The model under review builds one solid part; all positions refer to its coordinate system, in mm. Face numbers are marked on the shaded views. Coordinates: 2 decimals unless noted, no trailing zeros. Loops run counter-clockwise (first coordinate to the right, second up) from the corner with the lowest first, then second, coordinate; pieces in that order, holes last. Notation, with made-up numbers: M 32.5,-35 L 68.5,-35 A14 cw 68.5,-11 Z; hole C 2,38 d2. An arc over 180 degrees is marked long. Use one line per item in the form item = value.
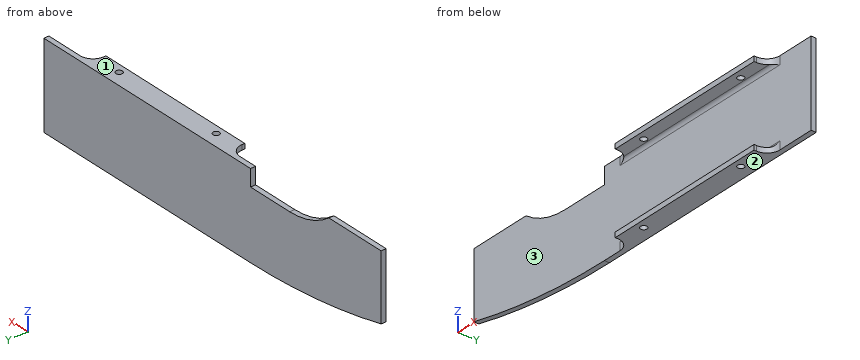
```python
from build123d import *

# Parameters (mm, degrees)
SKETCH1_W           = 132.917449813
SKETCH1_H           = 12
SKETCH1_R           = 2.55
BOSS_EXTRUDE1_DEPTH = 4
SKETCH2_W           = 197.917449813
SKETCH2_H           = 67
BOSS_EXTRUDE2_DEPTH = 4
BOSS_EXTRUDE3_START = 4
SKETCH3_W           = 132.917449813
SKETCH3_H           = 12
SKETCH3_R           = 2.55
BOSS_EXTRUDE3_DEPTH = 4
FILLET1_R           = 10
FILLET2_R           = 2.5
BOSS_EXTRUDE4_DEPTH = 4


with BuildPart() as part:
    # Sketch1 → Boss-Extrude1 (new body)
    with BuildSketch(Plane.XY):
        with Locations((-116.458724907, 49.8)):
            Rectangle(SKETCH1_W, SKETCH1_H)
        with Locations((-162.917449813, 49.8)):
            Circle(SKETCH1_R, mode=Mode.SUBTRACT)
        with Locations((-70, 49.8)):
            Circle(SKETCH1_R, mode=Mode.SUBTRACT)
    extrude(amount=BOSS_EXTRUDE1_DEPTH)

    # Sketch2 → Boss-Extrude2 (add)
    with BuildSketch(Plane(origin=(0, 55.8, 0), x_dir=(1, 0, 0), z_dir=(0, 1, 0))):
        with Locations((-108.958724907, -33.5)):
            Rectangle(SKETCH2_W, SKETCH2_H)
    extrude(amount=BOSS_EXTRUDE2_DEPTH)

    # Sketch3 → Boss-Extrude3 (add)
    with BuildSketch(Plane(origin=(0, 0, 67), x_dir=(-1, 0, 0), z_dir=(0, 0, -1)).offset(BOSS_EXTRUDE3_START)):
        with Locations((116.458724907, 49.8)):
            Rectangle(SKETCH3_W, SKETCH3_H)
        with Locations(Location((162.917449813, 49.8, 0), (0, 0, 180))):
            Circle(SKETCH3_R, mode=Mode.SUBTRACT)
        with Locations(Location((70, 49.8, 0), (0, 0, 180))):
            Circle(SKETCH3_R, mode=Mode.SUBTRACT)
    extrude(amount=-BOSS_EXTRUDE3_DEPTH)

    # Fillet1
    fillet1_edges = [part.edges().sort_by_distance(p)[0] for p in [
        (-182.917449813, 55.8, 65),
        (-50, 55.8, 65),
        (-182.917449813, 55.8, 2),
        (-50, 55.8, 2),
    ]]
    fillet(fillet1_edges, radius=FILLET1_R)

    # Fillet2
    fillet2_edges = [part.edges().sort_by_distance(p)[0] for p in [
        (-116.458724906, 55.8, 4),
        (-116.458724906, 55.8, 63),
    ]]
    fillet(fillet2_edges, radius=FILLET2_R)

    # Sketch4 → Boss-Extrude4 (add)
    with BuildSketch(Plane(origin=(0, 59.8, 0), x_dir=(1, 0, 0), z_dir=(0, 1, 0))):
        with BuildLine():
            Line((-207.917449813, -53.837484988), (-207.917449813, 0))
            ThreePointArc((-207.917449813, 0), (-270.865841373, -3.763403666), (-332.917449813, -15))
            Line((-332.917449813, -15), (-332.917449813, -67))
            Line((-332.917449813, -67), (-282.917449813, -67))
            ThreePointArc((-282.917449813, -67), (-265.288923094, -57.223665565), (-245.417449813, -53.837484988))
            Line((-245.417449813, -53.837484988), (-207.917449813, -53.837484988))
        make_face()
    extrude(amount=-BOSS_EXTRUDE4_DEPTH)


solid = part.part
```
1. Add section B-B (x = -124). State the section outline as (y, z) points, then the cut area to 3 significant figures.
Response values:
outline = M 43.8,0 L 59.8,0 L 59.8,67 L 43.8,67 L 43.8,63 L 53.3,63 A2.5 cw 55.8,60.5 L 55.8,6.5 A2.5 cw 53.3,4 L 43.8,4 Z
area = 367 mm^2
2. Wall thickness on line 1 along Z through (x, y) = (-50, 53.5); line 2 along X through (y, z) = (49.8, 65.75); line 3 along Y through (x, z) = (-70, 1.6): over which ranges is each line inside the solid? List them lowest first. Write a range as from..to.
Response values:
line_1 = 0..4.01, 62.99..67
line_2 = -183.75..-165.47, -160.37..-72.55, -67.45..-49.17
line_3 = 43.8..47.25, 52.35..59.8
3. Add section D-D (x = -212.5). State the section outline as (y, z) points, then the cut area to 3 significant figures.
Response values:
outline = M 55.8,0.02 L 59.8,0.02 L 59.8,53.84 L 55.8,53.84 Z
area = 215 mm^2
4. Insertion check: P1, Ø0.6, axis at y = 44.5, z = 65.5, coming from the -X side; P2, Ø2, axis at x = -218, y = 58.5, coming from the +Z side; P3, Ø3, axis at x = -70, y = 49.8, coming from the +Z side; P4, Ø0.6, axis at y = 45, z = 66, coming from the +X side. Each pin has a flat end and moves straight along its axis. Give the tip position at first contact, or say it passes through.
Response values:
P1 = -182.92
P2 = 53.84
P3 = through
P4 = -50
5. The part is to be moulded in two halves that separate along Z. For the marked faces 1, 2 and 3, say which applies: pulls with the +Z half, pulls with the -Z half, needs draft (parallel to the pull), parting line crosses it, or undercut.
Response values:
face_1 = pulls with the +Z half
face_2 = pulls with the -Z half
face_3 = undercut
6. Add section A-A (y = 49.8). State the section outline as (x, z) points, then the cut area to 3 significant figures.
Response values:
outline = M -183.75,0 L -165.47,0 L -165.47,4 L -183.75,4 Z; M -183.75,63 L -165.47,63 L -165.47,67 L -183.75,67 Z; M -160.37,0 L -72.55,0 L -72.55,4 L -160.37,4 Z; M -160.37,63 L -72.55,63 L -72.55,67 L -160.37,67 Z; M -67.45,0 L -49.17,0 L -49.17,4 L -67.45,4 Z; M -67.45,63 L -49.17,63 L -49.17,67 L -67.45,67 Z
area = 995 mm^2
7. Add section C-C (z = 39). State the section outline as (x, y) points, then the cut area to 3 significant figures.
Response values:
outline = M -332.92,55.8 L -10,55.8 L -10,59.8 L -332.92,59.8 Z
area = 1,290 mm^2
